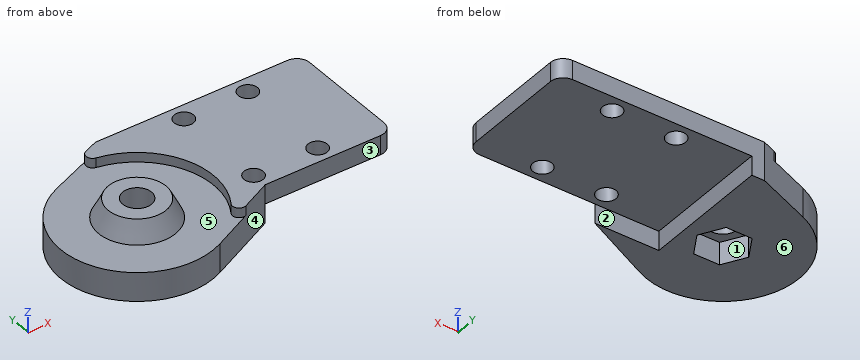
Autodesk Inventor part; units mm, degrees
ref_plane "Work Plane1" through (0, 0, 1.35) normal (0, 0, 1) x (1, 0, 0)
ref_plane "YZ Plane" through (0, 0, 0) normal (1, 0, 0) x (0, 1, 0)
ref_plane "XZ Plane" through (0, 0, 0) normal (0, 1, 0) x (-1, 0, 0)
sketch "Sketch1" plane through (0, 0, 0) normal (0, 0, 1) x (1, 0, 0)
  line L0 (-15, -10) -> (15, -10)
  line L1 (15, -10) -> (15, 10)
  line L2 (15, 10) -> (-15, 10)
  line L3 (-15, 10) -> (-15, -10)
  line L4 (-15, -10) -> (15, 10) construction
  line L5 (15, -10) -> (-15, 10) construction
  point P0 (0, 0)
  dimension "d0" = 30
  dimension "d1" = 20
extrude "Extrusion1" add sketch "Sketch1" along normal blind 3
sketch "Sketch2" plane through (0, 0, 3) normal (0, 0, 1) x (1, 0, 0)
  line L0 (-5, -7.5) -> (5, -7.5)
  line L1 (5, -7.5) -> (5, 7.5)
  line L2 (5, 7.5) -> (-5, 7.5)
  line L3 (-5, 7.5) -> (-5, -7.5)
  line L4 (-5, -7.5) -> (5, 7.5) construction
  line L5 (5, -7.5) -> (-5, 7.5) construction
  point P0 (0, 0)
  point P1 (0, 0)
  dimension "d4" = 10
  dimension "d5" = 15
hole "Hole1" at (-5, 7.5, 3) at (5, 7.5, 3) at (-5, -7.5, 3) at (5, -7.5, 3) direction (0, 0, -1) diameter 3 end through all
sketch "Sketch3" plane through (0, 0, 3) normal (0, 0, 1) x (1, 0, 0)
  line L0 (-18.979274, -1) -> (-16.958548, -4.5)
  line L1 (-16.958548, -4.5) -> (-18.979274, -8)
  line L2 (-18.979274, -8) -> (-23.020726, -8)
  line L3 (-23.020726, -8) -> (-25.041452, -4.5)
  line L4 (-25.041452, -4.5) -> (-23.020726, -1)
  line L5 (-23.020726, -1) -> (-18.979274, -1)
  circle A0 centre (-21, -4.5) radius 11.90625
  line L6 (15, -10) -> (15, 10)
  line L7 (15, 10) -> (-15, 10)
  line L8 (-15, 10) -> (-15, -10)
  line L9 (-15, -10) -> (15, -10)
  line L10 (-100, -4.5) -> (100, -4.5) construction
  line L11 (100, -4.5) -> (100, 4.5) construction
  line L12 (100, 4.5) -> (-100, 4.5) construction
  line L13 (-100, 4.5) -> (-100, -4.5) construction
  line L14 (-100, -4.5) -> (100, 4.5) construction
  line L15 (100, -4.5) -> (-100, 4.5) construction
  line L16 (-15, 10) -> (-17, 10)
  line L17 (-17, 10) -> (-25.507677, 6.519965)
  line L18 (15, -10) -> (15, -12)
  line L19 (15, -12) -> (-19.52358, -16.314354)
  line L20 (-22.587713, -1.75) -> (-19.412287, -1.75) construction
  line L21 (-19.412287, -1.75) -> (-17.824574, -4.5) construction
  line L22 (-17.824574, -4.5) -> (-19.412287, -7.25) construction
  line L23 (-19.412287, -7.25) -> (-22.587713, -7.25) construction
  line L24 (-22.587713, -7.25) -> (-24.175426, -4.5) construction
  line L25 (-24.175426, -4.5) -> (-22.587713, -1.75) construction
  circle A1 centre (-21, -4.5) radius 2 construction
  circle A2 centre (-21, -4.5) radius 1.5 construction
  line L26 (-5, -10) -> (-15.826239, -15.223385)
  point P0 (0, 0)
  point P1 (-21, -1)
  point P2 (-17.377304, -15.841731)
  point P3 (-10.440228, -10)
  point P4 (-15, 5.783909)
  point P5 (15, -11)
  dimension "d13" = 7
  dimension "d14" = 23.8125
  dimension "d15" = 9
  dimension "d16" = 200
  dimension "d19" = 4.5
  dimension "d30" = 21
  dimension "d44" = 2
  dimension "d46" = 5.5
  dimension "d47" = 4
  dimension "d48" = 0
  dimension "d49" = 3
  dimension "d73" = 20
extrude "Extrusion2" add sketch "Sketch3" against normal up to surface (3 mm away) contours L0 L1 L2 L3 L4 L5 | A0 L8 L9 | L17 L16 L8 A0 | A0 L9 L8 | A0 L9 L26
sketch "Sketch4" plane through (0, 0, 0) normal (0, 0, -1) x (-1, 0, 0)
  line L0 (-15, -10) -> (-15, 10)
  arc A0 (15.826239, -15.223385) -> (25.507677, 6.519965) centre (21, -4.5) ccw
  line L1 (-15, 10) -> (17, 10)
  line L2 (15, -10) -> (-15, -10)
  line L3 (-15, -10) -> (-15, 10)
  line L4 (-15, 10) -> (15, 10)
  line L5 (15, 10) -> (15, -10)
  line L6 (15, -10) -> (-15, 10) construction
  line L7 (-15, -10) -> (15, 10) construction
  line L8 (25.507677, 6.519965) -> (17, 10)
  line L9 (5, -10) -> (15.826239, -15.223385)
  line L10 (5, -10) -> (-15, -10)
  point P0 (0, 0)
  point P1 (15, 1.283909)
  point P2 (9.135819, -10)
extrude "Extrusion3" add sketch "Sketch4" along normal blind 3 contours L2 L5 L1 L8 A0 L9
sketch "Sketch5" plane through (0, 0, -3) normal (0, 0, -1) x (-1, 0, 0)
  arc A0 (15.826239, -15.223385) -> (25.507677, 6.519965) centre (21, -4.5) ccw
  line L0 (15, -10) -> (5, -10)
  line L1 (15, -5) -> (32.895747, -5)
  line L2 (100, -4.5) -> (-100, -4.5) construction
  line L3 (17, 10) -> (15, 10)
  line L4 (25.507677, 6.519965) -> (17, 10)
  line L5 (5, -10) -> (15.826239, -15.223385)
  line L6 (15, 10) -> (15, -10)
  point P0 (0, 0)
  dimension "d25" = 0.5
extrude "Extrusion4" add sketch "Sketch5" along normal blind 6
extrude "Extrusion5" cut sketch "Sketch3" against normal blind 1.5 contours L0 L1 L2 L3 L4 L5 | A0 L8 L9 | A0 L9 L8
fillet "Fillet1" radius 1 2 edges at (-25.5077, 6.52, 2.25) (-15.8262, -15.2234, 2.25)
sketch "Sketch6" plane through (0, 0, 1.5) normal (0, 0, 1) x (1, 0, 0)
  arc A0 (-25.507677, 6.519965) -> (-15.826239, -15.223385) centre (-21, -4.5) ccw
  arc A1 (-10.894095, -10.795194) -> (-18.916677, 7.222566) centre (-21, -4.5) ccw
  arc A2 (-19.120298, 9.1327) -> (-18.916677, 7.222566) centre (-18.7417, 8.207139) ccw
  line L0 (-19.120298, 9.1327) -> (-25.507677, 6.519965)
  line L1 (-15.826239, -15.223385) -> (-9.610763, -12.224576)
  arc A3 (-10.894095, -10.795194) -> (-9.610763, -12.224576) centre (-10.045305, -11.323924) ccw
  point P0 (0, 0)
hole "Hole2" at (-21, -4.5, 1.5) direction (0, 0, -1) diameter 4.5 depth 4
sketch "Sketch7" plane through (0, 0, -9) normal (0, 0, -1) x (-1, 0, 0)
  arc A0 (15.826239, -15.223385) -> (25.507677, 6.519965) centre (21, -4.5) ccw
  line L0 (15, -10) -> (5, -10)
  line L1 (18.979274, -1) -> (23.020726, -1)
  line L2 (23.020726, -1) -> (25.041452, -4.5)
  line L3 (25.041452, -4.5) -> (23.020726, -8)
  line L4 (23.020726, -8) -> (18.979274, -8)
  line L5 (18.979274, -8) -> (16.958548, -4.5)
  line L6 (16.958548, -4.5) -> (18.979274, -1)
  line L7 (25.507677, 6.519965) -> (17, 10)
  line L8 (17, 10) -> (15, 10)
  line L9 (5, -10) -> (15.826239, -15.223385)
  line L10 (15, 10) -> (15, -10)
  point P0 (0, 0)
  point P1 (21, -8)
  dimension "d39" = 7
extrude "Extrusion6" cut sketch "Sketch7" against normal blind 4 contours L9 L0 L10 L8 L7 A0 | L1 L2 L3 L4 L5 L6
sketch "Sketch9" plane through (0, 0, -5) normal (0, 0, -1) x (-1, 0, 0)
  arc A0 (15.826239, -15.223385) -> (25.507677, 6.519965) centre (21, -4.5) ccw
  circle A1 centre (21, -7) radius 6
  line L0 (27, -7) -> (27, -5)
  line L1 (15, -7) -> (15, -5)
  line L2 (15, -10) -> (15.803848, -10)
  line L3 (15, 10) -> (17, 10)
  line L4 (15.826239, -15.223385) -> (5, -10)
  line L5 (17, 10) -> (25.507677, 6.519965)
  line L6 (15, -10) -> (15, 10)
  line L7 (5, -10) -> (15, -10)
  point P0 (0, 0)
  dimension "d52" = 12
extrude "Extrusion8" [suppressed]
chamfer "Chamfer1" [suppressed]
sketch "Sketch11" plane through (0, 0, 1.5) normal (0, 0, 1) x (1, 0, 0)
  circle A0 centre (-21, -4.5) radius 2.25
  arc A1 (-25.507677, 6.519965) -> (-15.826239, -15.223385) centre (-21, -4.5) ccw
  arc A2 (-10.894095, -10.795194) -> (-18.916677, 7.222566) centre (-21, -4.5) ccw
  arc A3 (-19.120298, 9.1327) -> (-18.916677, 7.222566) centre (-18.7417, 8.207139) ccw
  line L0 (-19.120298, 9.1327) -> (-25.507677, 6.519965)
  circle A4 centre (-21, -4.5) radius 4.5
  line L1 (-15.826239, -15.223385) -> (-9.610763, -12.224576)
  arc A5 (-10.894095, -10.795194) -> (-9.610763, -12.224576) centre (-10.045305, -11.323924) ccw
  point P0 (0, 0)
  dimension "d61" = 9
extrude "Extrusion10" add sketch "Sketch11" along normal blind 3 contours A4
chamfer "Chamfer2" distance 1.5 distance2 3 1 edges at (-25.5, -4.5, 1.5) measured on face at (-15.1038, -11.5542, 1.5)
sketch "Sketch12" plane through (0, 0, -5) normal (0, 0, -1) x (-1, 0, 0)
  circle A0 centre (21, -4.5) radius 4.5
  line L0 (23.020726, -8) -> (18.979274, -8)
  line L1 (18.979274, -8) -> (16.958548, -4.5)
  line L2 (16.958548, -4.5) -> (18.979274, -1)
  line L3 (18.979274, -1) -> (23.020726, -1)
  line L4 (23.020726, -1) -> (25.041452, -4.5)
  line L5 (25.041452, -4.5) -> (23.020726, -8)
  point P0 (0, 0)
  point P1 (21, -8)
  dimension "d67" = 7
extrude "Extrusion11" cut sketch "Sketch12" against normal blind 5.5 contours L0 L1 L2 L3 L4 L5
sketch "Sketch13" plane through (0, 0, -5) normal (0, 0, -1) x (-1, 0, 0)
  line L0 (25.041452, -4.5) -> (23.020726, -8)
  line L1 (23.020726, -8) -> (18.979274, -8)
  line L2 (18.979274, -8) -> (16.958548, -4.5)
  arc A0 (15.826239, -15.223385) -> (25.507677, 6.519965) centre (21, -4.5) ccw
  line L3 (25.041452, -7) -> (25.041452, -5)
  line L4 (16.958548, -7) -> (16.958548, -5)
  line L5 (18.979274, -1) -> (23.020726, -1)
  line L6 (23.020726, -1) -> (25.041452, -4.5)
  line L7 (16.958548, -4.5) -> (18.979274, -1)
  line L8 (15, 10) -> (17, 10)
  line L9 (15.826239, -15.223385) -> (5, -10)
  line L10 (17, 10) -> (25.507677, 6.519965)
  line L11 (15, -10) -> (15, 10)
  line L12 (5, -10) -> (15, -10)
  point P0 (0, 0)
extrude "Extrusion12" cut sketch "Sketch13" against normal up to surface (2 mm away)
ref_plane "Work Plane1" through (0, 0, 1.35) normal (0, 0, 1) x (1, 0, 0)
fillet "Fillet4" radius 2 2 edges at (15, -10, 1.5) (15, 10, 1.5)
properties part number "UpperCarriagePivotMount" material "ABS Plastic"
Input: part model. Units: mm. Frame: model coordinates. Face numbers are marked on the shaded views. A direction names the side the tool comes from. Coordinates: 2 decimals unless noted, no trailing zeros. Order: outer loops, then holes, each group sorted by start corner. A loop starts at its lowest first (then second) coordinate and runs counter-clockwise, first axis right, second up.
1. Ray query, line 1 along Y through (x, z) = (-5, 0.8); line 2 along X through (y, z) = (7.5, 1.9); line 3 along X through (y, z) = (-7.5, 1.85). Return the intervals inside material, ascending.
Checked values:
line 1: y = -10 to -9, -6 to 6, 9 to 10
line 2: x = -19.45 to -6.5, -3.5 to 3.5, 6.5 to 15
line 3: x = -25.99 to -16.01, -9.48 to -6.5, -3.5 to 3.5, 6.5 to 15
2. Cut plane B-B, the plane z = 2.5. Return loops of the section in (x, y), plus the area to 3 significant figures.
Checked values:
outline: circle Ø11 at (-21, -4.5); (-19.12, 9.13) arc R1 ccw to (-18.92, 7.22) arc R11.91 cw to (-10.89, -10.8) arc R1 ccw to (-9.61, -12.22) - (-5, -10) - (13, -10) arc R2 ccw to (15, -8) - (15, 8) arc R2 ccw to (13, 10) - (-17, 10) - close; hole circle Ø4.5 at (-21, -4.5); hole circle Ø3 at (-5, -7.5); hole circle Ø3 at (-5, 7.5); hole circle Ø3 at (5, -7.5); hole circle Ø3 at (5, 7.5)
area: 598 mm2
3. Cut plane D-D, the plane y = -7.25. Count the separate pieces of the cut face and the enclosed holes in it, plus the area to 3 significant figures.
Checked values:
separate pieces: 3
enclosed holes: 0
area: 153 mm2
4. Cut plane C-C, the plane x = -1. Return loops of the section in (y, z), plus the area to 3 significant figures.
Checked values:
outline: (-10, 0) - (10, 0) - (10, 3) - (-10, 3) - close
area: 60.0 mm2
5. Contact query for flat-ended pins moving along their axis: P1, Ø12, axis at x = -2, y = -11.5, coming from the -Z side; P2, Ø0.9, axis at x = 4.5, z = 2, coming from the -Y side; P3, Ø2, axis at x = 2, y = 5, coming from the +Z side; P4, Ø3, axis at x = -21, z = -1.5, coming from the +Y side. Output: stop coordinate, or through.
Checked values:
P1: stops at z = -3
P2: stops at y = -10
P3: stops at z = 3
P4: stops at y = 8.98
6. Draft query along X for the marked faces 4, 5 and 6. Return one class per face: +X half, -X half, draft (parallel to the pull), parting line (faces both ways), or undercut.
Checked values:
face 4: +X half
face 5: undercut
face 6: draft
7. Access query for the marked faces 1, 2 and 3. Directions: +Z, -Z, +X, -X, +Y, -Y. A direction counts if a zero-diameter tool reaches every point of the face in a straight line with its end or side. Return the directions, or none.
Checked values:
face 1: -Z
face 2: -Z, +X, +Y
face 3: +Z, -Z, +X, -Y
